Here's the drawing with two shaded views (mm, measured from the low corner). I have some questions. A direction names the side the tool comes from. Give positions to 0.01 mm unless a question says otherwise; leave off trailing zeros. Loops run counter-clockwise (first coordinate to the right, second up) from the corner with the lowest first, then second, coordinate; pieces in that order, holes last. Notation, with made-up numbers: (3, 19) - (37, 19) arc R10 ccw to (37, 28) - close; hole circle Ø3 at (89, 6). An arc over 180 degrees is marked (long way). Use a Markdown table: item, result. Add a question column.
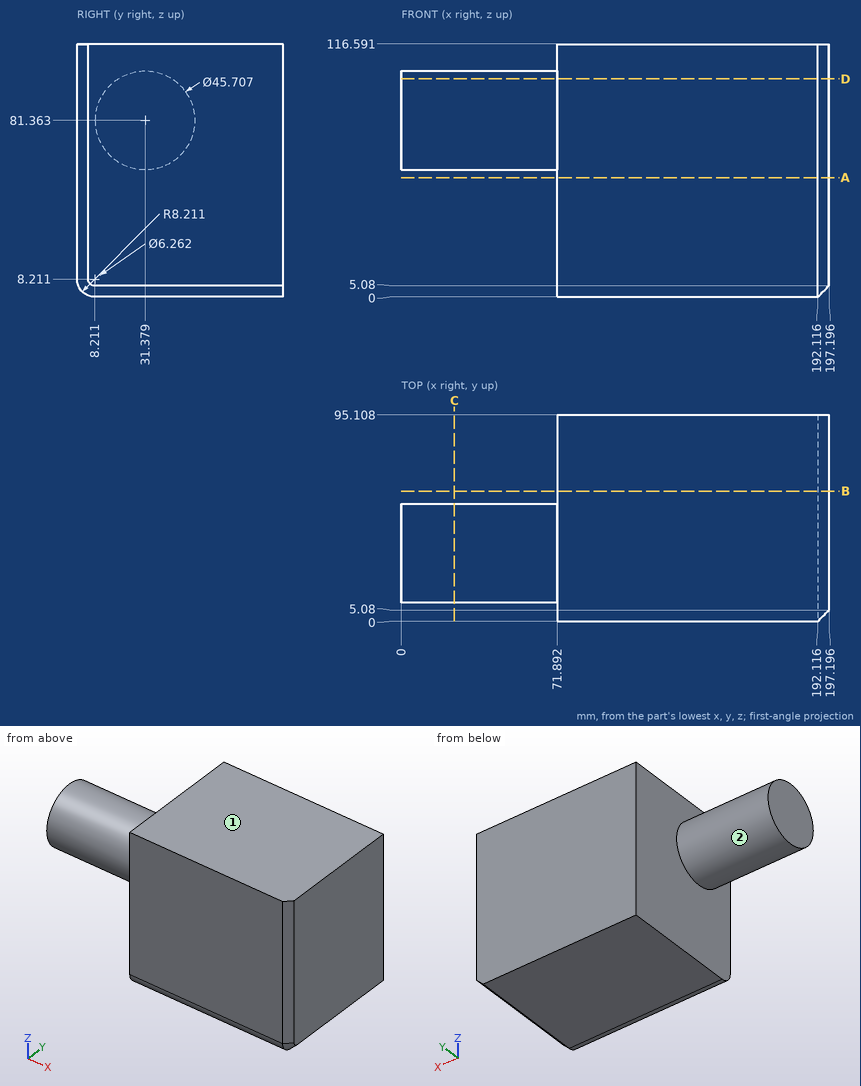
1. Please list where these lines run through material, in increasing order: line 1 along X through (y, z) = (9.5, 102.5) (1 decimal); line 2 along Z through (x, y) = (143.5, 8); line 3 along Z through (x, y) = (165.5, 5.5). Write a range as [from, to].
2. Suppose I cut it at B-B (y = 60). List the corners of the cut face in (x, z) for me (1 decimal).
3. Will these pins go through, and if not, where does the flat tip stop? P1, Ø5, axis at y = 68.5, z = 74, coming from the -X side; P2, Ø1, axis at x = 28.5, z = 71, coming from the -Y side.
4. Suppose I cut it at C-C (x = 24.5). List the corners of the cut face in (y, z) for me, and give its area (3 significant figures).
5. Suppose I cut it at A-A (z = 55). List the corners of the cut face in (x, y) for me (1 decimal), and give its area (3 significant figures).
6. On a 3-axis mill with a long thin cutter (end or side, diameter ignored), from which of +Z, -Z, +X, -X, +Y, -Y can I reach the whole of each face in a straight line? I mean the marked faces 1 and 2. Say none if no direction works.
7. Suppose I cut it at D-D (z = 100.5). List the corners of the cut face in (x, y) for me (1 decimal), and give its area (3 significant figures).
Results below:
| question | item | result |
|---|---|---|
| 1 | line 1 | [71.9, 197.2] |
| 1 | line 2 | [0, 116.59] |
| 1 | line 3 | [0.46, 116.59] |
| 2 | outline | (71.9, 0) - (192.1, 0) - (197.2, 5.1) - (197.2, 116.6) - (71.9, 116.6) - close |
| 3 | P1 | x = 71.89 |
| 3 | P2 | y = 10.76 |
| 4 | outline | circle Ø45.71 at (31.38, 81.36) |
| 4 | area | 1,640 mm² |
| 5 | outline | (71.9, 0) - (192.1, 0) - (197.2, 5.1) - (197.2, 95.1) - (71.9, 95.1) - close |
| 5 | area | 11,900 mm² |
| 6 | face 1 | +Z, +X, -X, +Y, -Y |
| 6 | face 2 | -X |
| 7 | outline | (0, 18.9) - (71.9, 18.9) - (71.9, 0) - (192.1, 0) - (197.2, 5.1) - (197.2, 95.1) - (71.9, 95.1) - (71.9, 43.9) - (0, 43.9) - close |
| 7 | area | 13,700 mm² |
